Geometry: final body of the model. Coordinates: model frame, mm. Face numbers are marked on the shaded views. A direction names the side the tool comes from. Give positions to 0.01 mm unless a question says otherwise; leave off trailing zeros. Loops run counter-clockwise (first coordinate to the right, second up) from the corner with the lowest first, then second, coordinate; pieces in that order, holes last. Notation, with made-up numbers: M 71,57 L 86,57 A20 cw 86,90 Z; hole C 9,80 d1. An arc over 180 degrees is marked long. One line per question, with ' | ' between items. Start each with the question number.
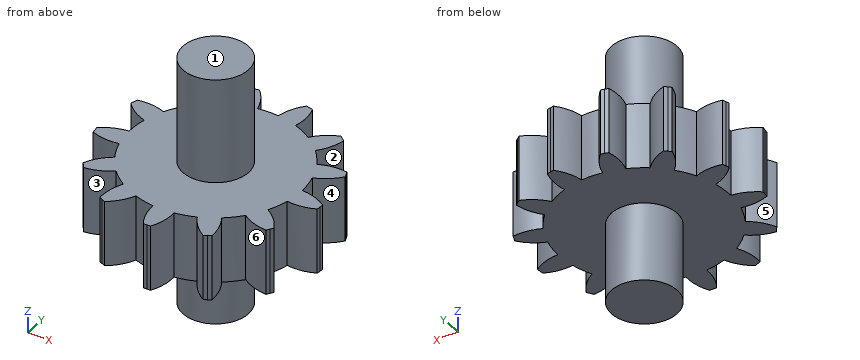
from build123d import *

# Parameters (mm, degrees)
F1_DEPTH      = 2.5
F2_R          = 1.25
F3_DEPTH      = 4
F3_DEPTH_BACK = 5.5


with BuildPart() as f1:
    # F0 (on Top) → F1 (new body)
    with BuildSketch(Plane.XY):
        with BuildLine():
            ThreePointArc((16.398417, 19.565806), (16.410022, 19.496985), (16.422997, 19.428409))
            ThreePointArc((16.422997, 19.428409), (16.944024, 19.308565), (17.477685, 19.340784))
            ThreePointArc((17.477685, 19.340784), (17.39318, 19.723361), (17.355326, 20.113326))
            ThreePointArc((17.355326, 20.113326), (16.837828, 19.979058), (16.379336, 19.704073))
            ThreePointArc((16.379336, 19.704073), (16.388187, 19.634844), (16.398417, 19.565806))
        make_face()
        with BuildLine():
            ThreePointArc((17.355326, 20.113326), (17.39318, 19.723361), (17.477685, 19.340784))
            ThreePointArc((17.477685, 19.340784), (17.608128, 18.969934), (17.782392, 18.617547))
            ThreePointArc((17.782392, 18.617547), (17.997136, 18.289841), (18.249753, 17.990357))
            ThreePointArc((18.249753, 17.990357), (18.537597, 17.722606), (18.855663, 17.491567))
            ThreePointArc((18.855663, 17.491567), (19.198102, 17.301194), (19.560961, 17.153412))
            ThreePointArc((19.560961, 17.153412), (19.940264, 17.050097), (20.329266, 16.993335))
            ThreePointArc((20.329266, 16.993335), (20.720951, 16.983908), (21.110925, 17.021682))
            ThreePointArc((21.110925, 17.021682), (21.494794, 17.106472), (21.865617, 17.23699))
            ThreePointArc((21.865617, 17.23699), (22.216818, 17.410668), (22.544568, 17.625345))
            ThreePointArc((22.544568, 17.625345), (22.845063, 17.878816), (23.112756, 18.166714))
            ThreePointArc((23.112756, 18.166714), (23.343017, 18.483709), (23.533459, 18.826109))
            ThreePointArc((23.533459, 18.826109), (23.681741, 19.190194), (23.784978, 19.569518))
            ThreePointArc((23.784978, 19.569518), (23.836075, 19.898895), (23.853167, 20.231773))
            ThreePointArc((23.853167, 20.231773), (23.85264, 20.290343), (23.851056, 20.348894))
            ThreePointArc((23.851056, 20.348894), (23.813154, 20.740185), (23.728286, 21.124037))
            ThreePointArc((23.728286, 21.124037), (23.598207, 21.493611), (23.424601, 21.844848))
            ThreePointArc((23.424601, 21.844848), (23.209199, 22.173705), (22.955667, 22.474148))
            ThreePointArc((22.955667, 22.474148), (22.668738, 22.74094), (22.351789, 22.971266))
            ThreePointArc((22.351789, 22.971266), (22.008233, 23.162351), (21.644118, 23.310558))
            ThreePointArc((21.644118, 23.310558), (21.266071, 23.413448), (20.87839, 23.470098))
            ThreePointArc((20.87839, 23.470098), (20.485383, 23.479638), (20.094101, 23.441656))
            ThreePointArc((20.094101, 23.441656), (19.711541, 23.357073), (19.34194, 23.22707))
            ThreePointArc((19.34194, 23.22707), (18.989517, 23.052878), (18.660704, 22.837408))
            ThreePointArc((18.660704, 22.837408), (18.361272, 22.584729), (18.094422, 22.297855))
            ThreePointArc((18.094422, 22.297855), (17.863318, 21.979836), (17.672302, 21.636241))
            ThreePointArc((17.672302, 21.636241), (17.524594, 21.273352), (17.421627, 20.895325))
            ThreePointArc((17.421627, 20.895325), (17.364786, 20.506335), (17.355326, 20.113326))
        make_face()
        with BuildLine():
            ThreePointArc((18.249753, 17.990357), (17.997136, 18.289841), (17.782392, 18.617547))
            ThreePointArc((17.782392, 18.617547), (17.386568, 18.258165), (17.108384, 17.801605))
            ThreePointArc((17.108384, 17.801605), (17.148394, 17.74442), (17.189536, 17.688044))
            ThreePointArc((17.189536, 17.688044), (17.231794, 17.632499), (17.275152, 17.577808))
            ThreePointArc((17.275152, 17.577808), (17.792193, 17.713824), (18.249753, 17.990357))
        make_face()
        with BuildLine():
            ThreePointArc((16.528468, 21.463052), (16.934121, 21.114802), (17.421627, 20.895325))
            ThreePointArc((17.421627, 20.895325), (17.524594, 21.273352), (17.672302, 21.636241))
            ThreePointArc((17.672302, 21.636241), (17.151683, 21.757845), (16.617916, 21.72743))
            ThreePointArc((16.617916, 21.72743), (16.593581, 21.662018), (16.570556, 21.596133))
            ThreePointArc((16.570556, 21.596133), (16.548849, 21.529802), (16.528468, 21.463052))
        make_face()
        with BuildLine():
            ThreePointArc((19.560961, 17.153412), (19.198102, 17.301194), (18.855663, 17.491567))
            ThreePointArc((18.855663, 17.491567), (18.672191, 16.989401), (18.638046, 16.45586))
            ThreePointArc((18.638046, 16.45586), (18.700048, 16.423818), (18.762677, 16.393019))
            ThreePointArc((18.762677, 16.393019), (18.825908, 16.363475), (18.889715, 16.335197))
            ThreePointArc((18.889715, 16.335197), (19.284322, 16.695915), (19.560961, 17.153412))
        make_face()
        with BuildLine():
            ThreePointArc((17.567404, 23.215623), (17.764752, 22.718747), (18.094422, 22.297855))
            ThreePointArc((18.094422, 22.297855), (18.361272, 22.584729), (18.660704, 22.837408))
            ThreePointArc((18.660704, 22.837408), (18.256231, 23.187028), (17.769469, 23.40815))
            ThreePointArc((17.769469, 23.40815), (17.717523, 23.361539), (17.666517, 23.313902))
            ThreePointArc((17.666517, 23.313902), (17.616471, 23.265257), (17.567404, 23.215623))
        make_face()
        with BuildLine():
            ThreePointArc((21.110925, 17.021682), (20.720951, 16.983908), (20.329266, 16.993335))
            ThreePointArc((20.329266, 16.993335), (20.400178, 16.463426), (20.617893, 15.97513))
            ThreePointArc((20.617893, 15.97513), (20.687684, 15.975573), (20.757452, 15.977407))
            ThreePointArc((20.757452, 15.977407), (20.82717, 15.980631), (20.896809, 15.985245))
            ThreePointArc((20.896809, 15.985245), (21.078583, 16.488028), (21.110925, 17.021682))
        make_face()
        with BuildLine():
            ThreePointArc((19.301797, 24.284631), (19.24563, 23.752956), (19.34194, 23.22707))
            ThreePointArc((19.34194, 23.22707), (19.711541, 23.357073), (20.094101, 23.441656))
            ThreePointArc((20.094101, 23.441656), (19.898434, 23.939197), (19.570188, 24.361201))
            ThreePointArc((19.570188, 24.361201), (19.502531, 24.344069), (19.435229, 24.325592))
            ThreePointArc((19.435229, 24.325592), (19.368309, 24.305777), (19.301797, 24.284631))
        make_face()
        with BuildLine():
            ThreePointArc((22.544568, 17.625345), (22.216818, 17.410668), (21.865617, 17.23699))
            ThreePointArc((21.865617, 17.23699), (22.174667, 16.800734), (22.594367, 16.469547))
            ThreePointArc((22.594367, 16.469547), (22.655958, 16.502372), (22.716882, 16.536418))
            ThreePointArc((22.716882, 16.536418), (22.777116, 16.571673), (22.836634, 16.608122))
            ThreePointArc((22.836634, 16.608122), (22.763932, 17.137788), (22.544568, 17.625345))
        make_face()
        with BuildLine():
            ThreePointArc((21.334318, 24.425177), (21.037503, 23.980505), (20.87839, 23.470098))
            ThreePointArc((20.87839, 23.470098), (21.266071, 23.413448), (21.644118, 23.310558))
            ThreePointArc((21.644118, 23.310558), (21.702083, 23.84204), (21.607551, 24.368249))
            ThreePointArc((21.607551, 24.368249), (21.539682, 24.384522), (21.471502, 24.399438))
            ThreePointArc((21.471502, 24.399438), (21.403039, 24.412991), (21.334318, 24.425177))
        make_face()
        with BuildLine():
            ThreePointArc((23.533459, 18.826109), (23.343017, 18.483709), (23.112756, 18.166714))
            ThreePointArc((23.112756, 18.166714), (23.589145, 17.924051), (24.11468, 17.825843))
            ThreePointArc((24.11468, 17.825843), (24.153962, 17.883531), (24.192086, 17.941991))
            ThreePointArc((24.192086, 17.941991), (24.229036, 18.0012), (24.264799, 18.061133))
            ThreePointArc((24.264799, 18.061133), (23.954275, 18.496343), (23.533459, 18.826109))
        make_face()
        with BuildLine():
            ThreePointArc((23.199342, 23.605065), (22.729875, 23.349265), (22.351789, 22.971266))
            ThreePointArc((22.351789, 22.971266), (22.668738, 22.74094), (22.955667, 22.474148))
            ThreePointArc((22.955667, 22.474148), (23.253983, 22.917814), (23.414821, 23.42768))
            ThreePointArc((23.414821, 23.42768), (23.362289, 23.473629), (23.30885, 23.518521))
            ThreePointArc((23.30885, 23.518521), (23.254527, 23.562339), (23.199342, 23.605065))
        make_face()
        with BuildLine():
            ThreePointArc((23.853167, 20.231773), (23.836075, 19.898895), (23.784978, 19.569518))
            ThreePointArc((23.784978, 19.569518), (24.319571, 19.57604), (24.830549, 19.733309))
            ThreePointArc((24.830549, 19.733309), (24.838522, 19.802645), (24.845111, 19.872125))
            ThreePointArc((24.845111, 19.872125), (24.850314, 19.941724), (24.854127, 20.011412))
            ThreePointArc((24.854127, 20.011412), (24.376921, 20.252463), (23.851056, 20.348894))
            ThreePointArc((23.851056, 20.348894), (23.85264, 20.290343), (23.853167, 20.231773))
        make_face()
        with BuildLine():
            ThreePointArc((24.469612, 22.012172), (23.935045, 22.003844), (23.424601, 21.844848))
            ThreePointArc((23.424601, 21.844848), (23.598207, 21.493611), (23.728286, 21.124037))
            ThreePointArc((23.728286, 21.124037), (24.198614, 21.378249), (24.577975, 21.754968))
            ThreePointArc((24.577975, 21.754968), (24.552814, 21.820066), (24.526359, 21.884651))
            ThreePointArc((24.526359, 21.884651), (24.498621, 21.948694), (24.469612, 22.012172))
        make_face()
    extrude(amount=F1_DEPTH)

    # F2 (on face) → F3 (join, two sides)
    with BuildSketch(Plane.XY.offset(2.5)) as f3_sk:
        with Locations((20.603167, 20.231773)):
            Circle(F2_R)
    extrude(amount=F3_DEPTH)
    extrude(f3_sk.sketch, amount=-F3_DEPTH_BACK)


solid = f1.part
Q1. Section A-A, the plane y = 23.75. Output: boundary loops of the cut face in (x, z), plus the area to 3 significant figures.
Q2. Section B-B, the plane z = 5. Output: boundary loops of the cut face in (x, y).
Q3. Draft query along X for the marked faces 1, 2 and 3. Return one class per face: released by +X, released by -X, zero draft, split by the parting line, or undercut.
Q4. Material intervals for L1, parallel to Z at x = 17.5, y = 21; L2, parallel to Y at x = 21.5, z = 6; L3, parallel to X at y = 19.5, z = 3, sorted ascending.
Q5. Contact query for flat-ended pins moving along their axis: pin 1 (3 mm diameter, centred on y = 19, z = 3.5, fed in from +X); pin 2 (1 mm diameter, centred on y = 18, z = 0.5, fed in from -X); pin 3 (1.5 mm diameter, centred on x = 20, y = 17.5, fed in from -Z); pin 4 (2 mm diameter, centred on y = 18, z = -0.5, fed in from +X). Output: stop coordinate, or through.
Q6. Set-up query: the marked faces 4, 5 and 6. Return all of +Z, -Z, +X, -X, +Y, -Y with unobstructed straight access to the full face (end or side cutting, diameter ignored); none if empty.
Model answer:
1) outline: M 19.25,0 L 19.99,0 L 19.99,2.5 L 19.25,2.5 Z; M 20.95,0 L 21.7,0 L 21.7,2.5 L 20.95,2.5 Z | area: 3.76 mm^2
2) outline: C 20.6,20.23 d2.5
3) face 1: zero draft | face 2: released by +X | face 3: undercut
4) L1: z = 0 to 2.5 | L2: y = 19.36 to 21.1 | L3: x = 19.59 to 21.62
5) pin 1: stops at x = 24.85 | pin 2: stops at x = 17.11 | pin 3: stops at z = 0 | pin 4: stops at x = 24.26
6) face 4: +Z, -Z, +X | face 5: +Z, -Z, -X | face 6: +Z, -Z, -Y
